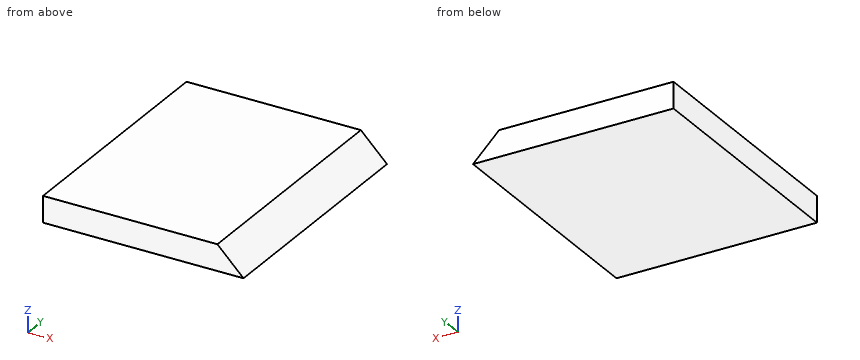
```python
from build123d import *

# Parameters (mm, degrees)
F0_W     = 76.7452418804
F0_H     = 92.9985865951
F1_DEPTH = 5
F3_SIZE  = 9.99999


# Not quite as in the source:
# - a fillet or chamfer is up to 0.001 mm smaller than in the source, because OpenCascade refuses the exact size


with BuildPart() as f1:
    # F0 (on Top) → F1 (new body, symmetric)
    with BuildSketch(Plane.XY):
        with Locations((38.3726209402, 46.4992932975)):
            Rectangle(F0_W, F0_H)
    extrude(amount=F1_DEPTH, both=True)

    # F3 (size 10 in the source; OpenCascade refuses exactly that, so slightly less here)
    f3_edges = [f1.edges().sort_by_distance(p)[0] for p in [
        (76.745242, 46.499293, 5),
    ]]
    chamfer(f3_edges, length=F3_SIZE)


solid = f1.part
```
Source: CAD feature listing. Evaluate the final solid. Frame: model axes, mm. Round coordinates to 2 decimals unless told otherwise and drop trailing zeros. Loops run counter-clockwise (first coordinate to the right, second up) from the corner with the lowest first, then second, coordinate; pieces in that order, holes last.
1. Ray query, L1, parallel to X at y = 51.5, z = -1.25; L2, parallel to X at y = 79, z = -0.25; L3, parallel to Z at x = 71.5, y = 78. Return the intervals inside material, ascending.
2. Section query C-C on x = 70. Output: boundary loops of the cut face in (y, z), and give its area (3 significant figures).
3. Section query B-B on z = -0.5. Output: boundary loops of the cut face in (x, y), and give its area (3 significant figures).
Answers below:
1. L1: x = 0 to 73
1. L2: x = 0 to 72
1. L3: z = -5 to 0.25
2. outline: (0, -5) - (93, -5) - (93, 1.75) - (0, 1.75) - close
2. area: 627 mm2
3. outline: (0, 0) - (72.25, 0) - (72.25, 93) - (0, 93) - close
3. area: 6,720 mm2
